The drawing under review shows one solid part. Ordinate dimensions are in mm from its lowest x, y, z. A direction names the side the tool comes from. Give positions to 0.01 mm unless a question says otherwise; leave off trailing zeros. Order: outer loops, then holes, each group sorted by start corner. A loop starts at its lowest first (then second) coordinate and runs counter-clockwise, first axis right, second up. Notation, with made-up numbers: M 64.25,-33 L 112.25,-33 A22 cw 112.25,-14 Z; hole C 14,25.25 d1. An arc over 180 degrees is marked long. Put each result on its own line as item: value. Start each with the question number.
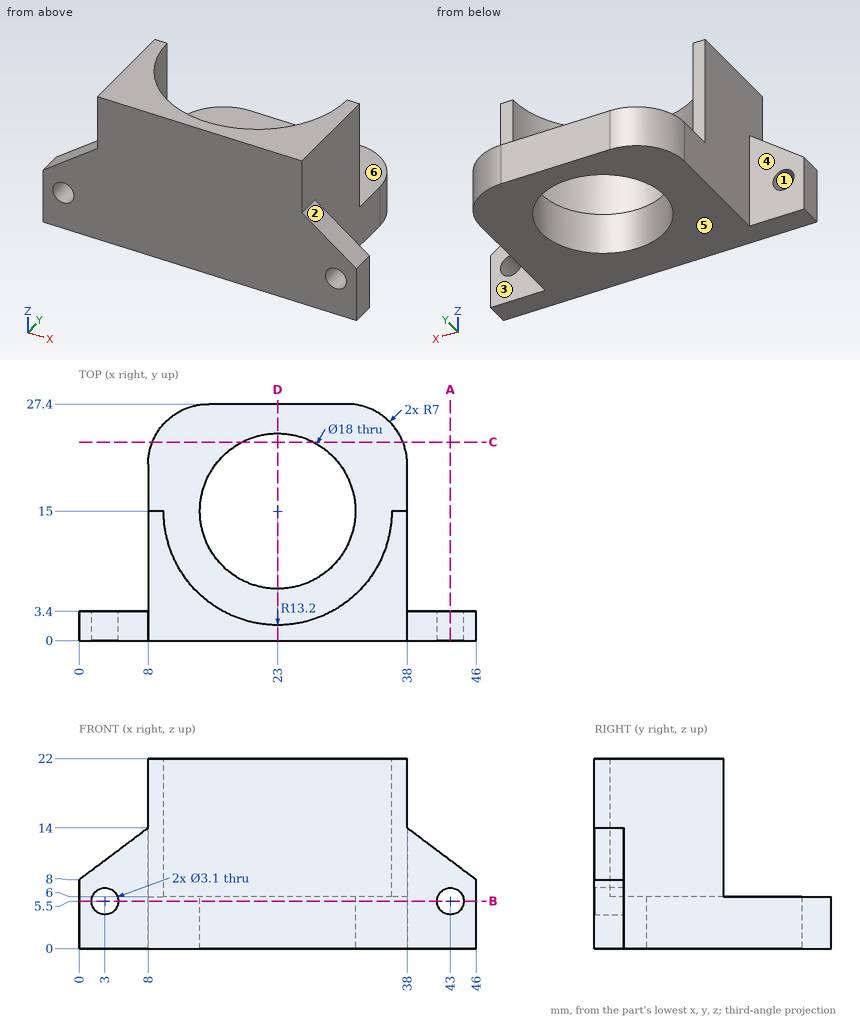
1. Consider section B-B on z = 5.5. Give the boundary of the cut face in (x, y).
2. Insertion check: pin 1 (3 mm diameter, centred on x = 3, z = 5.5, fed in from +Y); pin 2 (0.9 mm diameter, centred on x = 8.5, z = 11, fed in from +Y); pin 3 (2.5 mm diameter, centred on x = 43, z = 5, fed in from +Y); pin 4 (12 mm diameter, centred on y = 9.5, z = 11.5, fed in from -X). Each pin has a flat end and moves straight along its axis. Give the tip position at first contact, or say it passes through.
3. The part is to be moulded in two halves that separate along X. For the marked faces 1, 2 and 3, say which applies: +X half, -X half, draft (parallel to the pull), parting line (faces both ways), or undercut.
4. Consider section D-D on x = 23. Give the boundary of the cut face in (y, z), then the cut area to 3 significant figures.
5. Consider section A-A on x = 43. Give the boundary of the cut face in (y, z), then the cut area to 3 significant figures.
6. To check wall thickness, follow probe 1 along Y at (x, z) = (23, 2.65); probe 2 along X at (y, z) = (4.5, 19.25); probe 3 along X at (y, z) = (10.5, 3). State the ranges of each line that lie inside material, in increasing order.
7. Machinability: for the marked faces 4, 5 and 6, which of the approach directions +Z, -Z, +X, -X, +Y, -Y give a long, thin tool a straight path to every point of the face, cutting with its end or side? Answer none if there is none.
8. Consider section C-C on y = 23. Give the boundary of the cut face in (x, z).
Returned:
1. outline: M 0,0 L 1.45,0 L 1.45,3.4 L 0,3.4 Z; M 4.55,0 L 41.45,0 L 41.45,3.4 L 38,3.4 L 38,20.4 A7 ccw 31,27.4 L 15,27.4 A7 ccw 8,20.4 L 8,3.4 L 4.55,3.4 Z; M 44.55,0 L 46,0 L 46,3.4 L 44.55,3.4 Z; hole C 23,15 d18
2. pin 1: passes through
2. pin 2: stops at y = 15
2. pin 3: stops at y = 3.4
2. pin 4: stops at x = 8
3. face 1: undercut
3. face 2: +X half
3. face 3: draft
4. outline: M 0,0 L 6,0 L 6,6 L 1.8,6 L 1.8,22 L 0,22 Z; M 24,0 L 27.4,0 L 27.4,6 L 24,6 Z
4. area: 85.2 mm2
5. outline: M 0,0 L 3.4,0 L 3.4,3.95 L 0,3.95 Z; M 0,7.05 L 3.4,7.05 L 3.4,10.25 L 0,10.25 Z
5. area: 24.3 mm2
6. probe 1: y = 0 to 6, 24 to 27.4
6. probe 2: x = 8 to 15, 31 to 38
6. probe 3: x = 8 to 15.21, 30.79 to 38
7. face 4: +Z, -Z, -X, +Y
7. face 5: -Z, +X, -X, +Y, -Y
7. face 6: +Z, +Y
8. outline: M 8.5,0 L 18.88,0 L 18.88,6 L 8.5,6 Z; M 27.12,0 L 37.5,0 L 37.5,6 L 27.12,6 Z
